from build123d import *

# Parameters (mm, degrees)
SKETCH_1_W        = 9.6
SKETCH_1_H        = 9.6
EXTRUDE_1_DEPTH   = 4.5
SKETCH_3_R        = 0.25
EXTRUDE_3_DEPTH   = 4.5
SKETCH_4_R        = 1.1
EXTRUDE_1_2_DEPTH = 1.5


with BuildPart() as part:
    # 草图1 → Extrude 1 (new body)
    with BuildSketch(Plane(origin=(0, 0, 0), x_dir=(1, 0, 0), z_dir=(0, 1, 0))):
        Rectangle(SKETCH_1_W, SKETCH_1_H)
    extrude(amount=EXTRUDE_1_DEPTH)

    # 草图3 → 拉伸3 (add)
    with BuildSketch(Plane(origin=(0, 0, -4.8), x_dir=(-1, 0, 0), z_dir=(0, 0, -1))):
        with Locations(Location((0, 2.25, 0), (0, 0, 180))):
            Circle(SKETCH_3_R)
        with Locations(Location((2.595978382, 2.25, 0), (0, 0, 180))):
            Circle(SKETCH_3_R)
        with Locations(Location((-2.595978382, 2.25, 0), (0, 0, 180))):
            Circle(SKETCH_3_R)
    extrude(amount=EXTRUDE_3_DEPTH)

    # 草图4 → Extrude 1 2 (add)
    with BuildSketch(Plane.XY.offset(4.8)):
        with Locations(Location((-3.5, 3.2, 0), (0, 0, 180))):
            Circle(SKETCH_4_R)
    extrude(amount=EXTRUDE_1_2_DEPTH)


solid = part.part
Model file for the job. Use its own axes, mm. A direction names the side the tool comes from. Coordinates: 2 decimals unless noted, no trailing zeros. Order: outer loops, then holes, each group sorted by start corner. A loop starts at its lowest first (then second) coordinate and runs counter-clockwise, first axis right, second up. Notation, with made-up numbers: M -29,2 L 15,2 A18 cw 15,26 Z; hole C 11,24 d10. An arc over 180 degrees is marked long. Return JSON: item names as keys, results as strings.
1. Flat gauge pins, fed straight in: pin 1 (4 mm diameter, centred on x = 2, z = -2, fed in from -Y); pin 2 (1.5 mm diameter, centred on x = 1, y = 1, fed in from -Z). Where does each tip first touch, or does it go through?
Ans:
{"pin 1": "y = 0", "pin 2": "z = -4.8"}
2. Saw through at B-B (y = 3.2). Give the cut face in (x, z), and give its area (3 significant figures).
Ans:
{"outline": "M -4.8,-4.8 L 4.8,-4.8 L 4.8,4.8 L -2.4,4.8 L -2.4,6.3 L -4.6,6.3 L -4.6,4.8 L -4.8,4.8 Z", "area": "95.5 mm^2"}
3. Drill centre lines: probe 1 along Z at (x, y) = (-2.75, 2.5); probe 2 along Z at (x, y) = (1.5, 1.45); probe 3 along Y at (x, z) = (-3.25, 5.5). Where is each one in solid material? Low to high.
Ans:
{"probe 1": "-4.8 to 6.3", "probe 2": "-4.8 to 4.8", "probe 3": "2.13 to 4.27"}
4. Saw through at C-C (z = -5.5). Give the cut face in (x, y), and give its area (3 significant figures).
Ans:
{"outline": "C -2.6,2.25 d0.5; C 0,2.25 d0.5; C 2.6,2.25 d0.5", "area": "0.589 mm^2"}
5. Saw through at A-A (x = 0). Give the cut face in (y, z), and give its area (4 significant figures).
Ans:
{"outline": "M 0,-4.8 L 2,-4.8 L 2,-9.3 L 2.5,-9.3 L 2.5,-4.8 L 4.5,-4.8 L 4.5,4.8 L 0,4.8 Z", "area": "45.45 mm^2"}
6. Tool access for faces 1 (the face through (-4.09, 2.27, 5.54)), 2 (the face through (0, 4.5, 0)): list every direction of +Z, -Z, +X, -X, +Y, -Y with a clear straight run to the whole face (end or side of a thin tool).
Ans:
{"face 1": "+Z", "face 2": "+Z, -Z, +X, -X, +Y"}
7. Saw through at D-D (x = 3). Give the cut face in (y, z), and give its area (3 significant figures).
Ans:
{"outline": "M 0,-4.8 L 4.5,-4.8 L 4.5,4.8 L 0,4.8 Z", "area": "43.2 mm^2"}
